Geometry: see drawing. Coordinates: mm, zero at the bounding-box minimum. Coordinates: 2 decimals unless noted, no trailing zeros. Write each loop counter-clockwise with the first axis right and the second up, starting at its lowest first coordinate (ties: lowest second). Pieces come first, ordered by that corner, then holes.
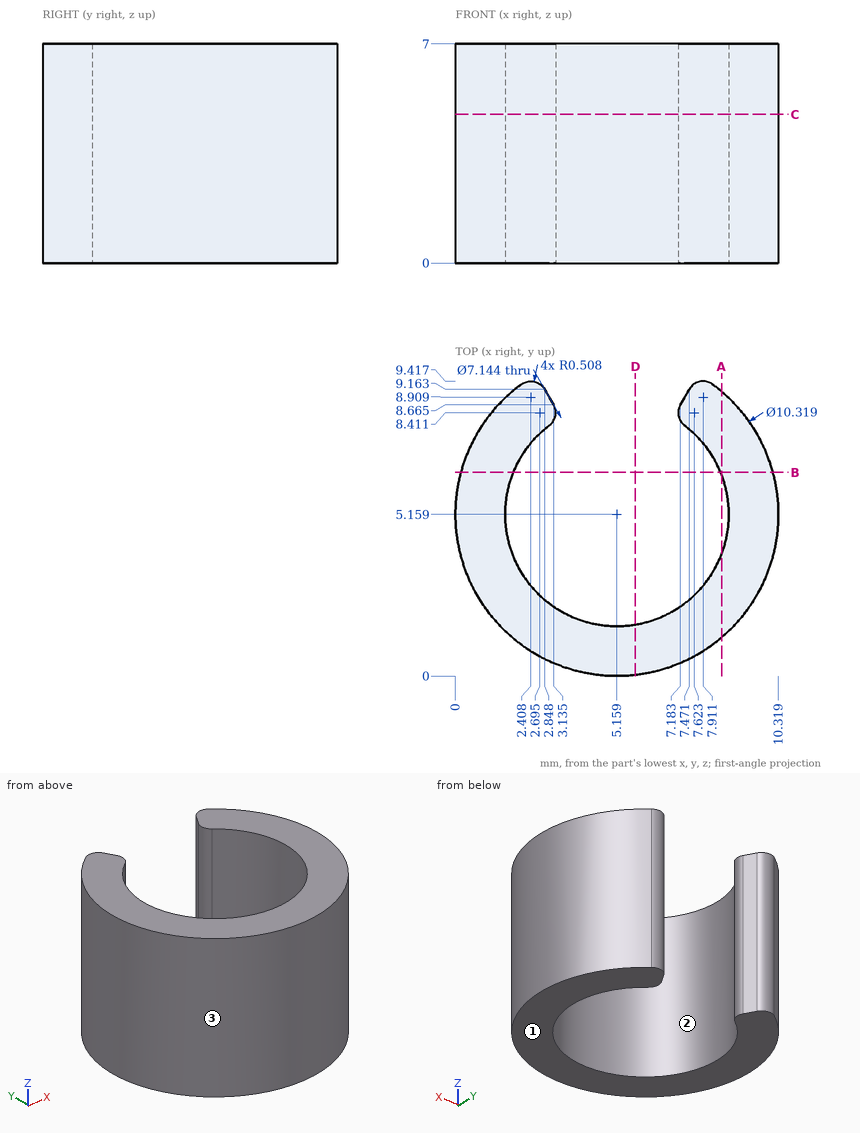
Item 1: Pin query (flat end, axial travel): pin 1 (1.5 mm diameter, centred on y = 4.5, z = 1, fed in from +X); pin 2 (1.5 mm diameter, centred on y = 7.5, z = 4.5, fed in from +X); pin 3 (1.5 mm diameter, centred on y = 1.5, z = 1, fed in from +X); pin 4 (3 mm diameter, centred on x = 2, z = 1.5, fed in from -Y) (1 decimal). Return the tip coordinate at first contact, or that it passes through.
Derived:
pin 1: stops at x = 10.32
pin 2: stops at x = 10.07
pin 3: stops at x = 9.42
pin 4: stops at y = 0.3
Item 2: Section B-B, the plane y = 6.5. Output: boundary loops of the cut face in (x, z), plus the area to 3 significant figures.
Derived:
outline: (0.18, 0) - (1.85, 0) - (1.85, 7) - (0.18, 7) - close; (8.47, 0) - (10.14, 0) - (10.14, 7) - (8.47, 7) - close
area: 23.4 mm2
Item 3: Section C-C, the plane z = 4.75. Output: boundary loops of the cut face in (x, y) (1 decimal).
Derived:
outline: (2.1, 9.3) arc R5.2 ccw (long way) to (8.2, 9.3) arc R0.5 ccw to (7.5, 9.2) - (7.2, 8.7) arc R0.5 ccw to (7.3, 8) arc R3.6 cw (long way) to (3, 8) arc R0.5 ccw to (3.1, 8.7) - (2.8, 9.2) arc R0.5 ccw to start
Item 4: Material intervals for probe 1 along Y at (x, z) = (2.25, 3.25) (1 decimal); probe 2 along Y at (x, z) = (7.5, 5) (1 decimal); probe 3 along X at (y, z) = (3.25, 2.5) (1 decimal), sorted ascending.
Derived:
probe 1: y = 0.9 to 3.1, 7.2 to 9.4
probe 2: y = 0.6 to 2.5, 7.9 to 9.2
probe 3: x = 0.4 to 2.1, 8.2 to 10
Item 5: Section D-D, the plane x = 5.75. Output: boundary loops of the cut face in (y, z).
Derived:
outline: (0.03, 0) - (1.64, 0) - (1.64, 7) - (0.03, 7) - close
Item 6: Pull-direction query (X, two-part tool) for the marked faces 1, 2 and 3; classes: released by +X, released by -X, zero draft, split by the parting line, or undercut.
Derived:
face 1: zero draft
face 2: undercut
face 3: split by the parting line
Item 7: Section A-A, the plane x = 8.5. Output: boundary loops of the cut face in (y, z) (1 decimal).
Derived:
outline: (1.2, 0) - (3.9, 0) - (3.9, 7) - (1.2, 7) - close; (6.4, 0) - (9.1, 0) - (9.1, 7) - (6.4, 7) - close
